Work out the finished part from the listing and answer in its coordinate system (mm). Face numbers are marked on the shaded views. A direction names the side the tool comes from. Coordinates: 2 decimals unless noted, no trailing zeros. Write each loop counter-clockwise with the first axis right and the second up, starting at its lowest first coordinate (ties: lowest second). Pieces come first, ordered by that corner, then holes. Notation, with made-up numbers: M -22.75,5.25 L -8.75,5.25 A20 cw -8.75,14.25 Z; hole C 79,35 d11. An arc over 180 degrees is marked long. Answer as CSV lines item,"result". Start each with the question number.
(1) A cutting plane is placed at D-D on x = 4.1. Give the vertices of the cut face in (y, z), then the cut area to 3 significant figures.
(2) The mould has two halves that part along Z. Classify the marked faces 1, 2 and 3: released by +Z, released by -Z, zero draft, split by the parting line, or undercut.
(3) A cutting plane is placed at C-C on z = -1.38. Give the vertices of the cut face in (x, y), then the cut area to 3 significant figures.
(4) A cutting plane is placed at B-B on y = 5.26. Give the vertices of the cut face in (x, z).
(5) A cutting plane is placed at A-A on x = 2.5. Give the vertices of the cut face in (y, z).
(6) Find the intervals of material crossed by L1, parallel to Z at x = 2.7, y = 5.26; L2, parallel to Z at x = 3, y = 5.26; L3, parallel to Y at x = 1.4, z = 3, in increasing order. Write a range as [from, to].
(7) Flat-ended cylindrical pins translate along their axes: P1, Ø3, axis at y = 3, z = 2, coming from the +X side; P2, Ø0.8, axis at x = 4, y = 1.5, coming from the +Z side; P3, Ø0.8, axis at x = 4, y = 4, coming from the -Z side. Find the tip coordinate at first contact, or state that the pin passes through.
(8) For the marked faces 4 and 5, determine the directions among +Z, -Z, +X, -X, +Y, -Y from which every point of the face is accessible in a straight line to the end or side of a thin tool.
Autodesk Inventor part; units mm, degrees
ref_plane "YZ Plane" through (0, 0, 0) normal (1, 0, 0) x (0, 1, 0)
ref_plane "XZ Plane" through (0, 0, 0) normal (0, 1, 0) x (-1, 0, 0)
ref_plane "XY Plane" through (0, 0, 0) normal (0, 0, 1) x (1, 0, 0)
sketch "Sketch1" plane through (0, 0, 0) normal (1, 0, 0) x (0, 1, 0)
  line L0 (0, 0) -> (6.5, 0)
  line L1 (6.5, 0) -> (6.5, -18)
  line L2 (6.5, -18) -> (0, -18)
  line L3 (0, -18) -> (0, 0)
  dimension "d0" = 6.5
  dimension "d1" = 18
extrude "Extrusion1" add sketch "Sketch1" along normal blind 2.75
sketch "Sketch2" plane through (2.75, 0, 0) normal (1, 0, 0) x (0, 0, -1)
  line L0 (0, 6.5) -> (0, 0)
  line L1 (0, 0) -> (18, 0)
  line L2 (0, 6.5) -> (3.3, 6.5)
  line L3 (3.3, 6.5) -> (3.3, 0)
  line L4 (3.3, 0) -> (0, 0)
  line L5 (0, 0) -> (0, 6.5)
  line L6 (18, 0) -> (18, 6.5)
  line L7 (18, 6.5) -> (0, 6.5)
  line L8 (18, 0) -> (14.7, 0)
  line L9 (14.7, 0) -> (14.7, 6.5)
  line L10 (14.7, 6.5) -> (18, 6.5)
  line L11 (18, 6.5) -> (18, 0)
  line L12 (3.3, 6.5) -> (14.7, 6.5)
  line L13 (14.7, 6.5) -> (14.7, 0)
  line L14 (14.7, 0) -> (3.3, 0)
  line L15 (3.3, 0) -> (3.3, 6.5)
  dimension "d4" = 3.3
  dimension "d5" = 3.3
extrude "Extrusion2" cut sketch "Sketch2" against normal blind 2.75 contours L7 L9 L1 L3
sketch "Sketch3" plane through (2.75, 0, 0) normal (1, 0, 0) x (0, 0, -1)
  line L0 (18, 6.5) -> (14.7, 6.5)
  line L1 (0, 0) -> (18, 0)
  line L2 (18, 0) -> (18, 6.5)
  line L3 (18, 6.5) -> (0, 6.5)
  line L4 (0, 6.5) -> (0, 0)
extrude "Extrusion3" add sketch "Sketch3" along normal blind 2
sketch "Sketch4" plane through (4.75, 0, 0) normal (1, 0, 0) x (0, 0, -1)
  line L0 (3.3, 6.5) -> (0, 6.5)
  line L1 (0, 6.5) -> (1.38, 6.5)
  line L2 (1.38, 6.5) -> (1.38, 5.26)
  line L3 (18, 6.5) -> (14.7, 6.5)
  line L4 (18, 6.5) -> (16.62, 6.5)
  line L5 (16.62, 6.5) -> (16.62, 5.26)
  circle A0 centre (1.38, 5.26) radius 0.7
  circle A1 centre (16.62, 5.26) radius 0.7
  point P0 (0, 0)
  dimension "d10" = 1.38
  dimension "d11" = 1.24
  dimension "d12" = 1.38
  dimension "d13" = 1.24
  dimension "d14" = 1.4
  dimension "d15" = 1.4
extrude "Extrusion4" cut sketch "Sketch4" against normal blind 20
sketch "Sketch5" plane through (0, 0, 0) normal (-1, 0, 0) x (0, 0, 1)
  line L0 (-18, 6.5) -> (0, 6.5)
  line L1 (0, 6.5) -> (6, 6.5)
  line L2 (6, 6.5) -> (6, 0)
  line L3 (6, 0) -> (0, 0)
  line L4 (0, 0) -> (0, 6.5)
  line L5 (-18, 0) -> (-18, 6.5)
  line L6 (-18, 6.5) -> (-24, 6.5)
  line L7 (-24, 6.5) -> (-24, 0)
  line L8 (-24, 0) -> (-18, 0)
  line L9 (-18, 0) -> (-18, 6.5)
  line L10 (-24, 3.25) -> (-21.5, 3.25)
  line L11 (-24, 6.5) -> (-24, 2.5)
  line L12 (-24, 2.5) -> (-21.5, 2.5)
  circle A0 centre (-21.5, 2.5) radius 1.5
  line L13 (6, 6.5) -> (6, 2.5)
  line L14 (6, 2.5) -> (3, 2.5)
  circle A1 centre (3, 2.5) radius 1.5
  point P0 (0, 0)
  dimension "d18" = 6
  dimension "d19" = 6.5
  dimension "d20" = 6
  dimension "d21" = 6.5
  dimension "d27" = 2.5
  dimension "d28" = 4
  dimension "d29" = 2.5
  dimension "d30" = 3
  dimension "d31" = 4
  dimension "d32" = 3
  dimension "d33" = 3
extrude "Extrusion6" add sketch "Sketch5" against normal blind 2 contours L1 L2 L3 L4 | L5 L8 L7 L12 A0 L10 L6 | L10 A0 L12 L7
properties part number "arduino_clamp"
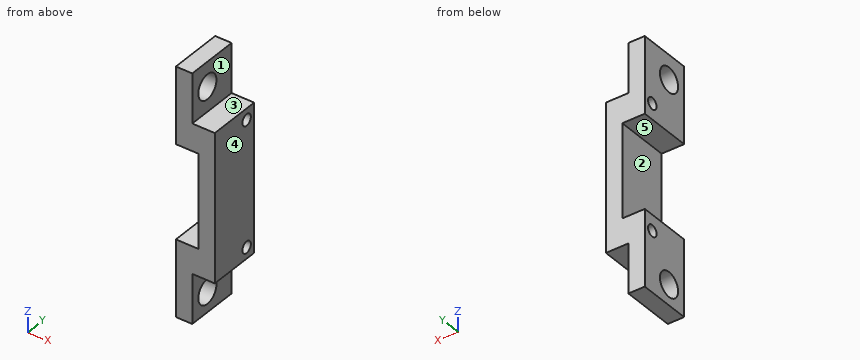
Here are the results:
1,outline,"M 0,-18 L 6.5,-18 L 6.5,0 L 0,0 Z; hole C 5.26,-16.62 d1.4; hole C 5.26,-1.38 d1.4"
1,area,"114 mm^2"
2,face 1,"zero draft"
2,face 2,"undercut"
2,face 3,"released by +Z"
3,outline,"M 0,0 L 4.75,0 L 4.75,4.56 L 0,4.56 Z; M 0,5.96 L 4.75,5.96 L 4.75,6.5 L 0,6.5 Z"
3,area,"24.2 mm^2"
4,outline,"M 0,-24 L 2,-24 L 2,-18 L 4.75,-18 L 4.75,-17.32 L 0,-17.32 Z; M 0,-15.92 L 4.75,-15.92 L 4.75,-2.08 L 0,-2.08 L 0,-3.3 L 2.75,-3.3 L 2.75,-14.7 L 0,-14.7 Z; M 0,-0.68 L 4.75,-0.68 L 4.75,0 L 2,0 L 2,6 L 0,6 Z"
5,outline,"M 0,-18 L 6.5,-18 L 6.5,-14.7 L 0,-14.7 Z; M 0,-3.3 L 6.5,-3.3 L 6.5,0 L 0,0 Z; hole C 5.26,-16.62 d1.4; hole C 5.26,-1.38 d1.4"
6,L1,"z = [-18, -17.32], [-15.92, -14.7], [-3.3, -2.08], [-0.68, 0]"
6,L2,"z = [-18, -17.32], [-15.92, -2.08], [-0.68, 0]"
6,L3,"y = [0, 1], [4, 6.5]"
7,P1,"stops at x = 2"
7,P2,"stops at z = 0"
7,P3,"stops at z = -18"
8,face 4,"+Z, -Z, +X, +Y, -Y"
8,face 5,"-X, +Y, -Y"
